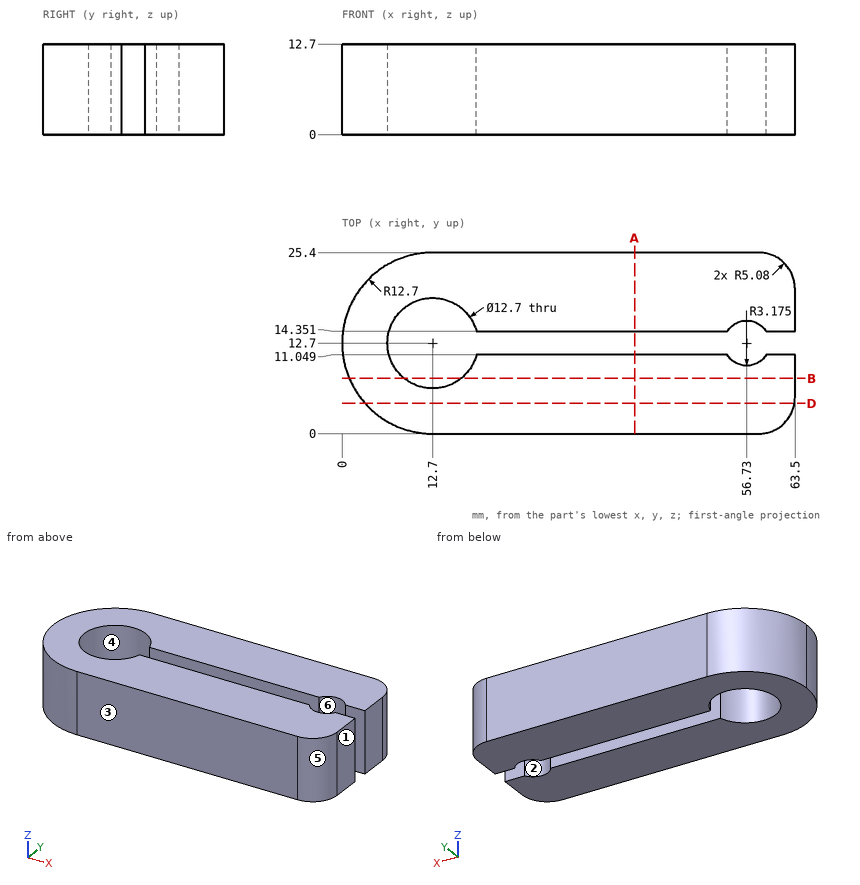
The figure shows three views and two pictorial views of one solid part (mm, origin at its lowest corner). Answer the questions. A direction names the side the tool comes from. Coordinates: 2 decimals unless noted, no trailing zeros. Loops run counter-clockwise (first coordinate to the right, second up) from the corner with the lowest first, then second, coordinate; pieces in that order, holes last. Notation, with made-up numbers: (48, -27) - (73, -27) arc R10 ccw to (73, -17) - close; hole circle Ø4 at (-32.75, -10). An arc over 180 degrees is marked (long way). Write item = value, one per line.
1) Find the intervals of material crossed by line 1 along Y through (x, z) = (38, 7); line 2 along Y through (x, z) = (12.7, 3.75); line 3 along X through (y, z) = (8.75, 9.5), in increasing order.
Responses:
line_1 = 0 to 11.05, 14.35 to 25.4
line_2 = 0 to 6.35, 19.05 to 25.4
line_3 = 0.63 to 7.73, 17.67 to 63.5
2) Section B-B (y = 7.75) is taken. Determine the outline of the cut face in (x, z), plus the area to 3 significant figures.
Responses:
outline = (1, 0) - (8.72, 0) - (8.72, 12.7) - (1, 12.7) - close; (16.68, 0) - (63.5, 0) - (63.5, 12.7) - (16.68, 12.7) - close
area = 693 mm^2
3) Section A-A (x = 41) is taken. Determine the outline of the cut face in (y, z).
Responses:
outline = (0, 0) - (11.05, 0) - (11.05, 12.7) - (0, 12.7) - close; (14.35, 0) - (25.4, 0) - (25.4, 12.7) - (14.35, 12.7) - close
4) Each of these flat-tipped pins is pushed along its axis until it touches: P1, Ø1, axis at y = 18, z = 8.5, coming from the -X side; P2, Ø3, axis at y = 16.5, z = 7.5, coming from the -X side; P3, Ø1.2, axis at x = 61, z = 6.5, coming from the -Y side. Where does it stop, or does it pass through?
Responses:
P1 = 0.94
P2 = 0.21
P3 = 0.4
5) Which of the six approach directions +Z, -Z, +X, -X, +Y, -Y give full straight-line access (tool end or side, diameter ignored) to the marked faces 5 and 6?
Responses:
face_5 = +Z, -Z, +X, -Y
face_6 = +Z, -Z
6) Section D-D (y = 4.25) is taken. Determine the outline of the cut face in (x, z).
Responses:
outline = (3.22, 0) - (63.43, 0) - (63.43, 12.7) - (3.22, 12.7) - close
7) Determine the mould class of the marked faces 1, 2, 3 and 4 for opening direction Y: pulls with the +Y half, pulls with the -Y half, needs draft (parallel to the pull), parting line crosses it, or undercut.
Responses:
face_1 = needs draft
face_2 = undercut
face_3 = pulls with the -Y half
face_4 = undercut
